Source: CAD feature listing. Evaluate the final solid. Frame: model axes, mm. Face numbers are marked on the shaded views. A direction names the side the tool comes from. Give positions to 0.01 mm unless a question says otherwise; leave off trailing zeros. Order: outer loops, then holes, each group sorted by start corner. A loop starts at its lowest first (then second) coordinate and runs counter-clockwise, first axis right, second up. Notation, with made-up numbers: (-24.75, -11) -> (24.25, -11) arc R28 ccw to (24.25, 9) -> close; hole circle Ø2 at (70, 5). An arc over 180 degrees is marked (long way). Use one line per item in the form item = value. Start each with the question number.
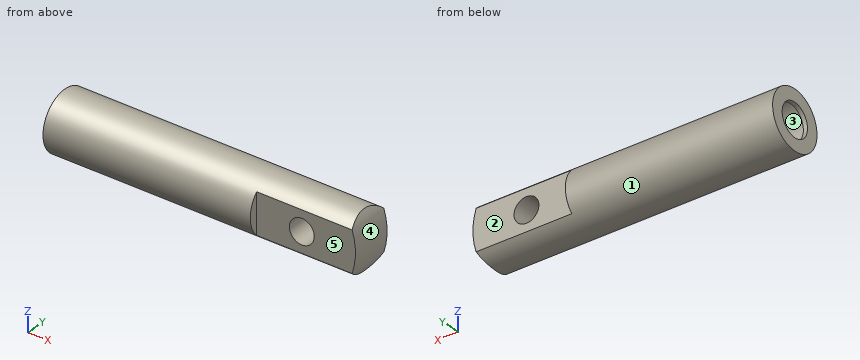
from build123d import *

# Parameters (mm, degrees)
SKETCH1_W           = 100
SKETCH1_H           = 2
BOSS_EXTRUDE1_START = -16
SKETCH2_R           = 12
BOSS_EXTRUDE1_DEPTH = 16
SKETCH3_R           = 31
BOSS_EXTRUDE2_DEPTH = 10
SKETCH4_OUTSIDE_W   = 96.516
SKETCH4_OUTSIDE_H   = 62.516
SKETCH4_OUTSIDE_R   = 14
CUT_EXTRUDE1_DEPTH  = 152.530264345
SKETCH5_R           = 6
CUT_EXTRUDE2_DEPTH  = 165.501660515
SKETCH6_R           = 12
SKETCH6_R_2         = 8
BOSS_EXTRUDE3_DEPTH = 2


with BuildPart() as part:
    # Sketch1 → Revolve1 (revolve)
    with BuildSketch(Plane(origin=(0, 0, 0), x_dir=(1, 0, 0), z_dir=(0, 1, 0))):
        with Locations((64.475, 13)):
            Rectangle(SKETCH1_W, SKETCH1_H)
    revolve(axis=Axis((134.425, 0, 0), (-1, 0, 0)))

    # Sketch2 → Boss-Extrude1 (add)
    with BuildSketch(Plane(origin=(114.475, 0, 0), x_dir=(0, 0, -1), z_dir=(1, 0, 0)).offset(BOSS_EXTRUDE1_START)):
        Circle(SKETCH2_R)
    extrude(amount=BOSS_EXTRUDE1_DEPTH)

    # Sketch3 → Boss-Extrude2 (add, symmetric)
    with BuildSketch(Plane(origin=(0, 0, 0), x_dir=(1, 0, 0), z_dir=(0, 1, 0))):
        with Locations((131.13820115, 0)):
            Circle(SKETCH3_R)
    extrude(amount=BOSS_EXTRUDE2_DEPTH, both=True)

    # Sketch4 outside → Cut-Extrude1 (cut, through all)
    with BuildSketch(Plane.ZY.offset(-14.475)):
        Rectangle(SKETCH4_OUTSIDE_W, SKETCH4_OUTSIDE_H)
        with Locations(Location((0, 0, 0), (0, 0, 180))):
            Circle(SKETCH4_OUTSIDE_R, mode=Mode.SUBTRACT)
    extrude(amount=-CUT_EXTRUDE1_DEPTH, mode=Mode.SUBTRACT)

    # Sketch5 → Cut-Extrude2 (cut, through all)
    with BuildSketch(Plane.XZ.offset(10)):
        with Locations(Location((136.284742261, 0, 0), (0, 0, 270))):
            Circle(SKETCH5_R)
    extrude(amount=-CUT_EXTRUDE2_DEPTH, mode=Mode.SUBTRACT)

    # Sketch6 → Boss-Extrude3 (add)
    with BuildSketch(Plane.ZY.offset(-14.475)):
        with Locations(Location((0, 0, 0), (0, 0, 180))):
            Circle(SKETCH6_R)
        Circle(SKETCH6_R_2, mode=Mode.SUBTRACT)
    extrude(amount=-BOSS_EXTRUDE3_DEPTH)


solid = part.part
1) Draft query along X for the marked faces 3, 4 and 5. Return one class per face: +X half, -X half, draft (parallel to the pull), parting line (faces both ways), or undercut.
2) Cut plane B-B, the plane y = -1.5. Return the cut outline in (x, z) (3 decimals).
3) Cut plane A-A, the plane z = 0. Return the cut outline in (x, y) (3 decimals).
4) Cut plane D-D, the plane x = 101.5. Return the cut outline in (y, z).
5) Reachability of the marked faces 1 and 2 from +Z, -Z, +X, -X, +Y, -Y: full face, straight path, thin tool, end or side. Return the list, or none.
6) Cut plane C-C, the plane x = 60. Return the cut outline in (y, z), plus the area to 3 significant figures.
7) Material intervals for probe 1 along X at (y, z) = (-5, 0) (3 decimals); probe 2 along Y at (x, z) = (40.5, 0); probe 3 along Y at (x, z) = (15.7, 0), sorted ascending.
8) Pin query (flat end, axial travel): pin 1 (8 mm diameter, centred on x = 127.5, z = 3, fed in from -Y); pin 2 (7 mm diameter, centred on y = -1.5, z = 3.5, fed in from +X); pin 3 (2 mm diameter, centred on y = -12.5, z = 0.5, fed in from +X) (3 decimals); pin 4 (3 mm diameter, centred on x = 122, z = -2, fed in from +Y). Return the tip coordinate at first contact, or that it passes through.
Output values:
q1.face_3 = undercut
q1.face_4 = +X half
q1.face_5 = draft
q2.outline = (14.475, -13.919) -> (158.837, -13.919) arc R31 ccw to (158.837, 13.919) -> (14.475, 13.919) -> (14.475, 7.858) -> (16.475, 7.858) -> (16.475, 11.906) -> (98.475, 11.906) -> (98.475, -11.906) -> (16.475, -11.906) -> (16.475, -7.858) -> (14.475, -7.858) -> close; hole circle Ø12 at (136.285, 0)
q3.outline = (14.475, -14) -> (114.475, -14) -> (114.475, -10) -> (130.285, -10) -> (130.285, 10) -> (114.475, 10) -> (114.475, 14) -> (14.475, 14) -> (14.475, 8) -> (16.475, 8) -> (16.475, 12) -> (98.475, 12) -> (98.475, -12) -> (16.475, -12) -> (16.475, -8) -> (14.475, -8) -> close; (142.285, -10) -> (162.138, -10) -> (162.138, 10) -> (142.285, 10) -> close
q4.outline = circle Ø28 at (0, 0)
q5.face_1 = +X, -X
q5.face_2 = +Z, -Z, +X, +Y
q6.outline = circle Ø28 at (0, 0); hole circle Ø24 at (0, 0)
q6.area = 163 mm^2
q7.probe_1 = 98.475 to 130.285, 142.285 to 162.138
q7.probe_2 = -14 to -12, 12 to 14
q7.probe_3 = -14 to -8, 8 to 14
q8.pin_1 = -10
q8.pin_2 = 162.14
q8.pin_3 = 114.475
q8.pin_4 = 10
